Print and shaded views of the part. All mm, measured from the part's lowest x, y and z. Give positions to 0.01 mm unless a question says otherwise; leave off trailing zeros. Write each loop counter-clockwise with the first axis right and the second up, starting at its lowest first coordinate (ties: lowest second). Pieces come first, ordered by that corner, then holes. Notation, with made-up numbers: (-11.75, 35) -> (9.25, 35) arc R33 cw to (9.25, 66) -> close; hole circle Ø10 at (-31.75, -5). An arc over 180 degrees is marked (long way). Put each result on its own line as item: value.
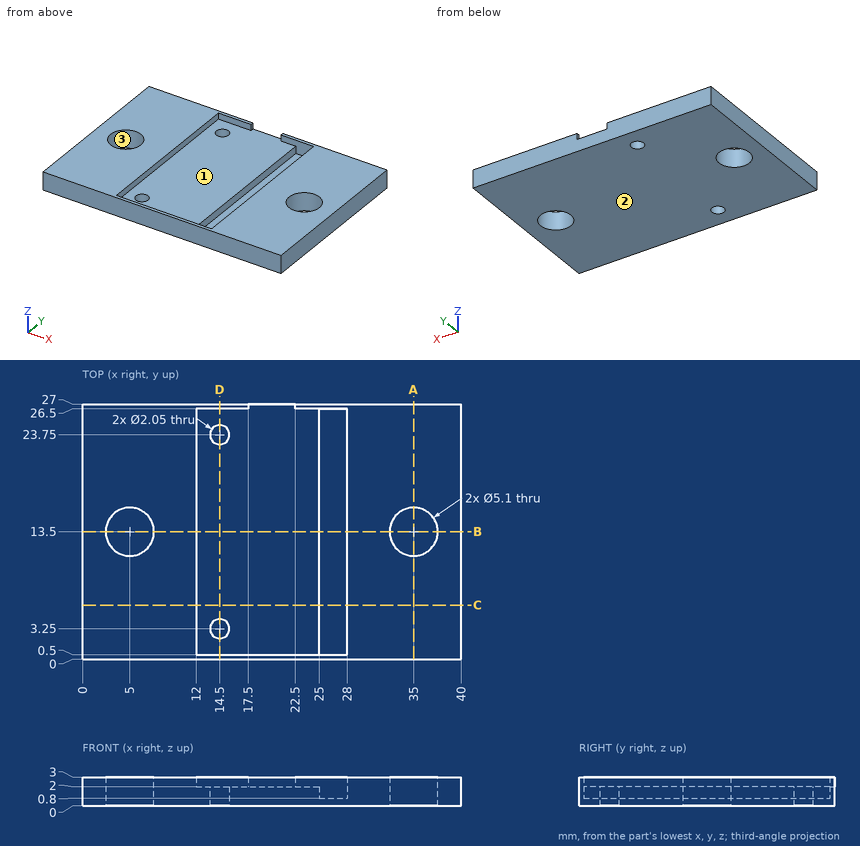
1) Slice it at C-C (y = 5.75). Write the cut outline in (x, z).
Filled sheet:
outline: (0, 0) -> (40, 0) -> (40, 3) -> (28, 3) -> (28, 0.8) -> (25, 0.8) -> (25, 2) -> (12, 2) -> (12, 3) -> (0, 3) -> close
2) Wall check: L1, parallel to Y at x = 14.5, z = 1.05 (3 decimals); L2, parallel to Y at x = 35, z = 1.3; L3, parallel to Y at x = 15, z = 1.05. Give the ranges that are in metal, low to high.
Filled sheet:
L1: 0 to 2.225, 4.275 to 22.725, 24.775 to 27
L2: 0 to 10.95, 16.05 to 27
L3: 0 to 2.36, 4.14 to 22.86, 24.64 to 27
3) Pull direction X, two halves, no side cores. Call the marked faces 1, 2 and 3: released by +X, released by -X, zero draft, split by the parting line, or undercut.
Filled sheet:
face 1: undercut
face 2: zero draft
face 3: undercut
4) Pin check, flat tip, straight feed: pin 1 (3.5 mm diameter, centred on x = 26, y = 8.5, fed in from +Z). Stop position of the tip, or through.
Filled sheet:
pin 1: z = 2
5) Slice it at B-B (y = 13.5). Write the cut outline in (x, z).
Filled sheet:
outline: (0, 0) -> (2.45, 0) -> (2.45, 3) -> (0, 3) -> close; (7.55, 0) -> (32.45, 0) -> (32.45, 3) -> (28, 3) -> (28, 0.8) -> (25, 0.8) -> (25, 2) -> (12, 2) -> (12, 3) -> (7.55, 3) -> close; (37.55, 0) -> (40, 0) -> (40, 3) -> (37.55, 3) -> close
6) Slice it at D-D (x = 14.5). Write the cut outline in (y, z) (3 decimals), plus the area to 3 significant figures.
Filled sheet:
outline: (0, 0) -> (2.225, 0) -> (2.225, 2) -> (0.5, 2) -> (0.5, 3) -> (0, 3) -> close; (4.275, 0) -> (22.725, 0) -> (22.725, 2) -> (4.275, 2) -> close; (24.775, 0) -> (27, 0) -> (27, 3) -> (26.5, 3) -> (26.5, 2) -> (24.775, 2) -> close
area: 46.8 mm2
7) Slice it at A-A (x = 35). Write the cut outline in (y, z), plus the area to 3 significant figures.
Filled sheet:
outline: (0, 0) -> (10.95, 0) -> (10.95, 3) -> (0, 3) -> close; (16.05, 0) -> (27, 0) -> (27, 3) -> (16.05, 3) -> close
area: 65.7 mm2
